Build history of the part. All positions in model axes, mm. A direction names the side the tool comes from. Coordinates: 2 decimals unless noted, no trailing zeros. Order: outer loops, then holes, each group sorted by start corner. A loop starts at its lowest first (then second) coordinate and runs counter-clockwise, first axis right, second up. Notation, with made-up numbers: (5.5, 22.5) - (58.5, 22.5) arc R17 cw to (58.5, 37.5) - close; hole circle Ø9 at (21, -2.75). An arc over 180 degrees is marked (long way). Answer as CSV lines item,"result". Start each with the question number.
Autodesk Inventor part; units mm, degrees
ref_plane "Work Plane1" through (29, 0, 0) normal (0, -1, 0) x (1, 0, 0)
ref_plane "YZ Plane" through (0, 0, 0) normal (1, 0, 0) x (0, 1, 0)
ref_plane "XZ Plane" through (0, 0, 0) normal (0, 1, 0) x (-1, 0, 0)
sketch "Esquisse1" plane through (0, 0, 0) normal (0, 0, 1) x (1, 0, 0)
  line L0 (-1.1667, 0) -> (8, 0)
  line L1 (8, 0) -> (8, 2.5)
  line L2 (8, 2.5) -> (2, 2.5)
  line L3 (2, 2.5) -> (1.5091, 2.5)
  line L4 (1.5091, 2.5) -> (0, 2.5)
  line L5 (0, 2.5) -> (0, 4.25)
  line L6 (0, 4.25) -> (-5, 4.25)
  line L7 (-5, 4.25) -> (-5, 2.3094)
  line L8 (-5, 2.3094) -> (-2.5, 2.3094)
  line L9 (-2.5, 2.3094) -> (-1.1667, 0)
  line L10 (-7.6, 0) -> (10.6, 0)
  line L11 (0, -0.85) -> (0, 5.1)
  line L12 (2, 2.5) -> (0, 2.5) construction
  dimension "d1" = 6
  dimension "d2" = 0.4909
  dimension "d3" = 5
  dimension "d4" = 2.5
  dimension "d5" = 60
  dimension "d6" = 5
  dimension "d7" = 5
  dimension "d8" = 4.6188
  dimension "d9" = 8.5
  dimension "d26" = 8
revolve "Corps" add sketch "Esquisse1" angle 360 about axis through (-1.1667, 0, 0) along (1, 0, 0)
sketch "Esquisse2" plane through (-5, 0, 0) normal (-1, 0, 0) x (0, 0, 1)
  circle A0 centre (0, 0) radius 2.3094
  line L0 (0, -5.95) -> (0, 5.95)
  line L1 (-5.95, 0) -> (5.95, 0)
  line L2 (2.3094, 0) -> (1.1547, -2)
  line L3 (1.1547, -2) -> (-1.1547, -2)
  line L4 (-1.1547, -2) -> (-2.3094, 0)
  line L5 (-2.3094, 0) -> (-1.1547, 2)
  line L6 (-1.1547, 2) -> (1.1547, 2)
  line L7 (1.1547, 2) -> (2.3094, 0)
extrude "Rainure" add sketch "Esquisse2" against normal up to next contours L7 A0 | A0 L2 | L6 L0 A0 | A0 L0 L3 | L0 L6 A0 | A0 L3 L0 | L4 A0 | A0 L5
fillet "Congé1" radius 0.5 1 edges at (-5, -4.25, 0)
thread "Filetage"
chamfer "Chanfrein1" distance 0.4908 distance2 0.4908 1 edges at (8, -2.5, 0) measured on face at (8, -0.6238, -0.819)
ref_plane "Work Plane1" through (29, 0, 0) normal (0, -1, 0) x (1, 0, 0)
fillet "Fillet2" radius 0.1 1 edges at (0, -2.5, 0)
equation "\"d30\" = R"
equation "\"d17\" = RR"
equation "\"d13\" = GEL"
equation "\"d15\" = -0.5 * SPD + 0.5 * GD"
equation "\"d16\" = GUL"
equation "\"d1\" = GEL"
equation "\"d3\" = KOH"
equation "\"d4\" = INTI"
equation "\"d6\" = GD"
equation "\"d7\" = BDM"
equation "\"d8\" = 1.1547 * SW"
equation "\"d9\" = KOD"
equation "\"d26\" = NLG"
equation "\"GD\" = 5"
equation "\"NLG\" = 8"
equation "\"GEL\" = 6"
equation "\"KOD\" = 8.5"
equation "\"KOH\" = 5"
equation "\"INTI\" = 2.5"
equation "\"GAL\" = 0.61345 * PTC"
equation "\"GUL\" = 0.61345 * PTC"
equation "\"BDM\" = NND"
equation "\"SW\" = 4"
equation "\"RR\" = 0.5"
equation "\"SPD\" = NND - 1.2269 * PTC"
equation "\"R\" = 0.1"
equation "\"TOA\" = 30deg"
equation "\"GD1\" = THREADDIA - 1.2269 * PTC"
equation "\"THREADDIA\" = 5"
equation "\"FAWI\" = 45deg"
equation "\"PTC\" = 0.8"
equation "\"NND\" = 5"
equation "\"E0\" = 1.155 * SW"
properties part number "ISO 4762 - M5 x 8" material "Acier inoxydable 440C"
(1) Band-saw the part on A-A on x = -3.75. List the corners of the cut face in (y, z).
(2) Which spindle directions (+Z, -Z, +X, -X, +Y, -Y) get a long thin tool onto all of the face, cutting with end or side? Do faces 1 (the flat face through (8, 0, 0)), 2 (the flat face through (-4, 2, 0)), 3 (the flat face through (0, 2, 2)). Say none if no direction does.
(3) Band-saw the part on B-B on x = 1. List the corners of the cut face in (y, z), plus the area to 3 significant figures.
(4) Probe L1, parallel to Y at x = -3.25, z = 0.5; L2, parallel to X at y = -1.5, z = -3.25; L3, parallel to Z at x = 2, y = -1.5. List the from-to ranges inside material, lowest first. Write a range as [from, to].
(5) Drop flat-ended pins along their axis: pin 1 Ø3 at (x, y) = (3, -0.5) entering from -Z; pin 2 Ø4 at (x, y) = (-1.5, 3) entering from +Z; pin 3 Ø3 at (x, z) = (3, -1) entering from -Y. Give the stop position or say it passes through.
(6) Pull direction Y, two halves, no side cores. Call faces 4 (the flat face through (-5, -2, 2)), 5 (the cylindrical face through (-2.282, 2.285, -3.584)), 6 (the flat face through (-3.679, 1.014, 1.724)): +Y half, -Y half, draft (parallel to the pull), parting line (faces both ways), or undercut.
Filled in:
1,outline,"circle Ø8.5 at (0, 0); hole (-2, -1.15) - (0, -2.31) - (2, -1.15) - (2, 1.15) - (0, 2.31) - (-2, 1.15) - close"
2,face 1,"+Z, -Z, +X, +Y, -Y"
2,face 2,"-X"
2,face 3,"+X"
3,outline,"circle Ø5 at (0, 0)"
3,area,"19.6 mm^2"
4,L1,"y = [-4.22, -2], [2, 4.22]"
4,L2,"x = [-5, 0]"
4,L3,"z = [-2, 2]"
5,pin 1,"stops at z = -2.5"
5,pin 2,"stops at z = 4.13"
5,pin 3,"stops at y = -2.5"
6,face 4,"draft"
6,face 5,"parting line"
6,face 6,"undercut"
